```python
from build123d import *

# Parameters (mm, degrees)
SKETCH_1_W               = 27
SKETCH_1_H               = 17
EXTRUDE_1_DEPTH          = 1
SKETCH_2_R               = 2.55
CUT_EXTRUDE_1_DEPTH      = 16.984367363
EXTRUDE_2_DEPTH          = 17
SKETCH_6_W               = 1.5
SKETCH_6_H               = 2
EXTRUDE_3_DEPTH          = 2
CHAMFER_1_SIZE           = 1
CUT_EXTRUDE_4_REACH      = 39.316
SKETCH_8_R               = 2
FILLET_1_R               = 3
SKETCH_9_W               = 7
SKETCH_9_H               = 13
EXTRUDE_4_DEPTH          = 1.5
SKETCH_7_R               = 1.35
CUT_EXTRUDE_5_DEPTH      = 10
CUT_EXTRUDE_6_REACH      = 41.373
FILLET_2_R               = 2.2
SKETCH_13_W              = 11.6
SKETCH_13_H              = 5.4
EXTRUDE_6_DEPTH          = 5.4
CUT_EXTRUDE_7_DEPTH      = 45.299097095
CUT_EXTRUDE_7_DEPTH_BACK = 45.299097095
SKETCH_14_OUTSIDE_W      = 46.85
SKETCH_14_OUTSIDE_H      = 49.25
SKETCH_14_OUTSIDE_W_2    = 27
SKETCH_14_OUTSIDE_H_2    = 6.9
EXTRUDE_7_DEPTH          = 3.5
EXTRUDE_7_DEPTH_BACK     = 10.5
SKETCH_16_W              = 5.6
SKETCH_16_H              = 1.5
SKETCH_16_W_2            = 4.4
SKETCH_16_W_3            = 12.2
EXTRUDE_8_DEPTH          = 2
EXTRUDE_9_DEPTH          = 2.5
CUT_EXTRUDE_8_REACH      = 55.893
SKETCH_18_W              = 5
SKETCH_18_H              = 9
EXTRUDE_START            = -1.5
SKETCH_19_R              = 3.726433752
SKETCH_19_R_2            = 1.35
SKETCH_19_W              = 24.8
SKETCH_19_H              = 1.288897449
EXTRUDE_10_DEPTH         = 1.5
FILLET_4_R               = 2


# Some blends are built 0.0001 mm under size
with BuildPart() as part:
    # 草图1 → 凸台-拉伸1 (new body)
    with BuildSketch(Plane.XY):
        Rectangle(SKETCH_1_W, SKETCH_1_H)
    extrude(amount=EXTRUDE_1_DEPTH)

    # 草图2 → 切除-拉伸1 (cut, through all)
    with BuildSketch(Plane.XY.offset(1)):
        with Locations((0, 4.125)):
            Circle(SKETCH_2_R)
        with Locations((0, -4.125)):
            Circle(SKETCH_2_R)
        with Locations((8.27, 4.125)):
            Circle(SKETCH_2_R)
        with Locations((8.27, -4.125)):
            Circle(SKETCH_2_R)
        with Locations((-8.27, 4.125)):
            Circle(SKETCH_2_R)
        with Locations((-8.27, -4.125)):
            Circle(SKETCH_2_R)
    extrude(amount=-CUT_EXTRUDE_1_DEPTH, mode=Mode.SUBTRACT)

    # 草图3 → 凸台-拉伸2 (add)
    with BuildSketch(Plane.XZ.offset(8.5)):
        Polygon((13.5, 0), (19, 0), (19, -28.5), (-13.5, -28.5), (-13.5, -30), (20.5, -30), (20.5, 1), (13.5, 1), align=None)
    extrude(amount=-EXTRUDE_2_DEPTH)

    # 草图6 → 凸台-拉伸3 (add, symmetric)
    with BuildSketch(Plane(origin=(0, 0, 0), x_dir=(1, 0, 0), z_dir=(0, 1, 0))):
        Polygon((19, 0), (19, 5), (14, 0), align=None)
        Polygon((19, 28.5), (14, 28.5), (19, 23.5), align=None)
        with Locations((18.25, 20)):
            Rectangle(SKETCH_6_W, SKETCH_6_H)
    extrude(amount=EXTRUDE_3_DEPTH, both=True)

    # 倒角1
    chamfer_1_edges = [part.edges().sort_by_distance(p)[0] for p in [
        (-13.5, 0, 0),
    ]]
    chamfer(chamfer_1_edges, length=CHAMFER_1_SIZE - 0.0001)  # a hair under: the kernel refuses the full size

    # 草图8 → 切除-拉伸4 (cut, up to next)
    with BuildSketch(Plane(origin=(0, 0, 0), x_dir=(-1, 0, 0), z_dir=(0, 0, -1)), mode=Mode.PRIVATE) as cut_extrude_4_sk1:
        Circle(SKETCH_8_R)
    cut_extrude_4_tool1 = extrude(cut_extrude_4_sk1.sketch, amount=-CUT_EXTRUDE_4_REACH, mode=Mode.PRIVATE) & part.part
    add(cut_extrude_4_tool1.solids().sort_by_distance((0, 0, 0))[0], mode=Mode.SUBTRACT)

    # 圆角1
    fillet_1_edges = [part.edges().sort_by_distance(p)[0] for p in [
        (20.5, 0, 1),
        (20.5, 0, -30),
        (19, 5.25, -28.5),
        (19, 5.25, 0),
        (19, -5.25, 0),
        (19, -5.25, -28.5),
    ]]
    fillet(fillet_1_edges, radius=FILLET_1_R)

    # 草图9 → 凸台-拉伸4 (add)
    with BuildSketch(Plane(origin=(0, 0, -30), x_dir=(-1, 0, 0), z_dir=(0, 0, -1))):
        with Locations((0, 6.5)):
            Rectangle(SKETCH_9_W, SKETCH_9_H)
    extrude(amount=-EXTRUDE_4_DEPTH)

    # 草图7 → 切除-拉伸5 (cut)
    with BuildSketch(Plane(origin=(0, 0, -30), x_dir=(-1, 0, 0), z_dir=(0, 0, -1))):
        with Locations((0, 10)):
            Circle(SKETCH_7_R)
        with Locations((-8.5, 2.7)):
            Circle(SKETCH_7_R)
        with Locations((8.5, 2.7)):
            Circle(SKETCH_7_R)
    extrude(amount=-CUT_EXTRUDE_5_DEPTH, mode=Mode.SUBTRACT)

    # 草图11 → 切除-拉伸6 (cut, up to next)
    with BuildSketch(Plane(origin=(0, 0, -30), x_dir=(-1, 0, 0), z_dir=(0, 0, -1)), mode=Mode.PRIVATE) as cut_extrude_6_sk1:
        with BuildLine():
            Line((13.5, -8.5), (13.5, 0))
            Line((13.5, 0), (-9, 0))
            ThreePointArc((-9, 0), (-15.01040764, -2.48959236), (-17.5, -8.5))
            Line((-17.5, -8.5), (13.5, -8.5))
        make_face()
    cut_extrude_6_tool1 = extrude(cut_extrude_6_sk1.sketch, amount=-CUT_EXTRUDE_6_REACH, mode=Mode.PRIVATE) & part.part
    add(cut_extrude_6_tool1.solids().sort_by_distance((1.149624, -4.397011, -30))[0], mode=Mode.SUBTRACT)

    # 圆角2
    fillet_2_edges = [part.edges().sort_by_distance(p)[0] for p in [
        (-3.5, 13, -29.25),
        (-3.5, 8.5, -29.25),
        (3.5, 13, -29.25),
        (3.5, 8.5, -29.25),
        (-13.5, 0, -29.25),
        (-13.5, 8.5, -29.25),
    ]]
    fillet(fillet_2_edges, radius=FILLET_2_R)

    # 草图13 → 凸台-拉伸6 (add)
    with BuildSketch(Plane(origin=(0, 0, -30), x_dir=(-1, 0, 0), z_dir=(0, 0, -1))):
        with Locations((0, 2.7)):
            Rectangle(SKETCH_13_W, SKETCH_13_H)
    extrude(amount=EXTRUDE_6_DEPTH)

    # 草图14 outside → 切除-拉伸7 (cut, two sides: drawn at the far end of the back side and taken through both)
    with BuildSketch(Plane(origin=(0, 8.5, 0), x_dir=(1, 0, 0), z_dir=(0, 1, 0)).offset(-CUT_EXTRUDE_7_DEPTH_BACK)):
        with Locations((3.5, 17.2)):
            Rectangle(SKETCH_14_OUTSIDE_W, SKETCH_14_OUTSIDE_H)
        with Locations((0, 31.95)):
            Rectangle(SKETCH_14_OUTSIDE_W_2, SKETCH_14_OUTSIDE_H_2, mode=Mode.SUBTRACT)
    extrude(amount=CUT_EXTRUDE_7_DEPTH + CUT_EXTRUDE_7_DEPTH_BACK, mode=Mode.SUBTRACT)

    # 草图15 → 凸台-拉伸7 (add, two sides: drawn at the far end of the back side and taken through both)
    with BuildSketch(Plane.XZ.offset(-EXTRUDE_7_DEPTH_BACK)):
        Polygon((-19.25, -14.25), (-19.25, -30), (-11.3, -30), (-11.3, -28.5), (-17.75, -28.5), (-17.75, -19.35), (-16.15, -19.35), (-16.15, -17.35), (-17.75, -17.35), (-17.75, -16.25), (-15.25, -16.25), (-15.25, -14.25), align=None)
        Polygon((17.75, -28.5), (13.5, -28.5), (13.5, -30), (19.25, -30), (19.25, -14.25), (15.25, -14.25), (15.25, -16.25), (17.75, -16.25), (17.75, -17.35), (16.15, -17.35), (16.15, -19.35), (17.75, -19.35), align=None)
    extrude(amount=EXTRUDE_7_DEPTH + EXTRUDE_7_DEPTH_BACK)

    # 草图16 → 凸台-拉伸8 (add)
    with BuildSketch(Plane(origin=(0, 8.5, 0), x_dir=(1, 0, 0), z_dir=(0, 1, 0))):
        with Locations((-8.5, 29.25)):
            Rectangle(SKETCH_16_W, SKETCH_16_H)
        with Locations((-3.5, 29.25)):
            Rectangle(SKETCH_16_W_2, SKETCH_16_H)
        with Locations((7.4, 29.25)):
            Rectangle(SKETCH_16_W_3, SKETCH_16_H)
    extrude(amount=EXTRUDE_8_DEPTH)

    # 草图17 → 凸台-拉伸9 (add, symmetric)
    with BuildSketch(Plane(origin=(0, 3.5, 0), x_dir=(-1, 0, 0), z_dir=(0, -1, 0))):
        Polygon((17.75, 25.275), (14.525, 28.5), (17.75, 28.5), align=None)
        Polygon((-17.75, 25.275), (-17.75, 28.5), (-14.525, 28.5), align=None)
    extrude(amount=EXTRUDE_9_DEPTH, both=True)

    # 草图18 → 切除-拉伸8 (cut, up to next)
    with BuildSketch(Plane.ZY.offset(19.25), mode=Mode.PRIVATE) as cut_extrude_8_sk1:
        with Locations((-19.85, 3.5)):
            Rectangle(SKETCH_18_W, SKETCH_18_H)
    cut_extrude_8_tool1 = extrude(cut_extrude_8_sk1.sketch, amount=-CUT_EXTRUDE_8_REACH, mode=Mode.PRIVATE) & part.part
    add(cut_extrude_8_tool1.solids().sort_by_distance((-19.25, 3.5, -19.85))[0], mode=Mode.SUBTRACT)

    # 草图19 → 凸台-拉伸10 (add)
    # profile 1 of 2: a face of its own
    with BuildSketch(Plane.XY.offset(-28.5).offset(EXTRUDE_START)):
        with Locations((0, 10)):
            Circle(SKETCH_19_R)
        with Locations((0, 10)):
            Circle(SKETCH_19_R_2, mode=Mode.SUBTRACT)
    # profile 2 of 2: a face of its own
    with BuildSketch(Plane.XY.offset(-28.5).offset(EXTRUDE_START)):
        with Locations((1.1, -0.644448725)):
            Rectangle(SKETCH_19_W, SKETCH_19_H)
    extrude(amount=EXTRUDE_10_DEPTH)

    # 圆角4
    # the kernel refuses this fillet: 2 mm, written as the material it adds along each edge
    with BuildSketch(Plane(origin=(-5.8, 5.4, -30), x_dir=(0, 1, 0), z_dir=(1, 0, 0))) as fillet_4_piece_1:
        with BuildLine():
            CenterArc((FILLET_4_R, -FILLET_4_R), FILLET_4_R, 90, 90)
            Line((0, -FILLET_4_R), (0, 0))
            Line((0, 0), (FILLET_4_R, 0))
        make_face()
    extrude(amount=11.6)
    with BuildSketch(Plane(origin=(13.5, -1.288897449, -28.5), x_dir=(0, -1, 0), z_dir=(0, 0, -1))) as fillet_4_piece_2:
        with BuildLine():
            CenterArc((FILLET_4_R, FILLET_4_R), FILLET_4_R, 180, 90)
            Line((0, FILLET_4_R), (0, 0))
            Line((0, 0), (FILLET_4_R, 0))
        make_face()
    extrude(amount=1.5)
    with BuildSketch(Plane(origin=(17.75, 1, -28.5), x_dir=(-1, 0, 0), z_dir=(0, 1, 0)), Plane(origin=(-17.75, 6, -28.5), x_dir=(1, 0, 0), z_dir=(0, -1, 0)), Plane(origin=(-17.75, 10.5, -28.5), x_dir=(1, 0, 0), z_dir=(0, -1, 0)), Plane(origin=(17.75, -3.5, -28.5), x_dir=(-1, 0, 0), z_dir=(0, 1, 0))) as fillet_4_piece_3:
        with BuildLine():
            CenterArc((FILLET_4_R, FILLET_4_R), FILLET_4_R, 180, 90)
            Line((0, FILLET_4_R), (0, 0))
            Line((0, 0), (FILLET_4_R, 0))
        make_face()
    extrude(amount=9.5)
    with BuildSketch(Plane(origin=(-3.692737265, 10.5, -28.5), x_dir=(-1, 0, 0), z_dir=(0, 0, -1))) as fillet_4_piece_4:
        with BuildLine():
            CenterArc((1.459159814, 2), FILLET_4_R, 205.88535786, 64.11464214)
            ThreePointArc((-0.340178937, 1.126856222), (-0.125315404, 0.576944648), (0, 0))
            Line((0, 0), (1.459159814, 0))
        make_face()
    extrude(amount=1.5)
    with BuildSketch(Plane(origin=(3.692737265, 10.5, -28.5), x_dir=(-0.28900142054358374, 0.9573286681823493, 0), z_dir=(0, 0, -1))) as fillet_4_piece_5:
        with BuildLine():
            CenterArc((1.492958077, 1.974898363), FILLET_4_R, 196.798181975, 64.11464214)
            Line((-0.421699259, 1.396895522), (0, 0))
            ThreePointArc((0, 0), (0.588541981, 0.046769794), (1.177083962, 0))
        make_face()
    extrude(amount=1.5)
    with BuildSketch(Plane(origin=(-5.8, 0, -30), x_dir=(0, -1, 0), z_dir=(1, 0, 0))) as fillet_4_piece_6:
        with BuildLine():
            CenterArc((2, 1.869313554), FILLET_4_R, 180, 69.172765444)
            Line((0, 1.869313554), (0, 0))
            Line((0, 0), (1.288897449, 0))
        make_face()
    extrude(amount=11.6)
    with BuildSketch(Plane(origin=(-11.3, -1.288897449, -30), x_dir=(1, 0, 0), z_dir=(0, 0, 1))) as fillet_4_piece_7:
        with BuildLine():
            CenterArc((FILLET_4_R, -FILLET_4_R), FILLET_4_R, 90, 90)
            Line((0, -FILLET_4_R), (0, 0))
            Line((0, 0), (FILLET_4_R, 0))
        make_face()
    extrude(amount=1.5)
    # the kernel refuses this fillet: 2 mm, written as the material it takes off along each edge
    with BuildSketch(Plane(origin=(19.25, 15.5, -30), x_dir=(-1, 0, 0), z_dir=(0, -1, 0))) as fillet_4_2_piece_1:
        with BuildLine():
            CenterArc((FILLET_4_R, -FILLET_4_R), FILLET_4_R, 90, 90)
            Line((0, -FILLET_4_R), (0, 0))
            Line((0, 0), (FILLET_4_R, 0))
        make_face()
    extrude(amount=24, mode=Mode.SUBTRACT)
    with BuildSketch(Plane(origin=(-19.25, 15.5, -30), x_dir=(1, 0, 0), z_dir=(0, -1, 0))) as fillet_4_2_piece_2:
        with BuildLine():
            CenterArc((FILLET_4_R, FILLET_4_R), FILLET_4_R, 180, 90)
            Line((0, FILLET_4_R), (0, 0))
            Line((0, 0), (FILLET_4_R, 0))
        make_face()
    extrude(amount=24, mode=Mode.SUBTRACT)


solid = part.part
```
Geometry: final body of the model. Coordinates: model frame, mm. A direction names the side the tool comes from. Coordinates: 2 decimals unless noted, no trailing zeros. Order: outer loops, then holes, each group sorted by start corner. A loop starts at its lowest first (then second) coordinate and runs counter-clockwise, first axis right, second up. Notation, with made-up numbers: (16.5, 53) -> (62.5, 53) arc R23 cw to (62.5, 86) -> close; hole circle Ø5 at (-6.5, -14.5). An arc over 180 degrees is marked (long way). Write each question's results on one line, items separated by ' | '. Start each with the question number.
1) First-contact query: pin 1 (2.5 mm diameter, centred on x = -17.5, z = -20, fed in from +Y); pin 2 (1 mm diameter, centred on x = -0.5, z = -33, fed in from +Y); pin 3 (1.8 mm diameter, centred on x = -16.5, y = -3, fed in from -Z). Flat tips, straight axial feed; report the tip coordinate or a pass-through.
2) Mould query, pull axis Z, two halves, no side actions, for faces 1 (the flat face through (17.75, 4, -23)), 2 (the flat face through (-4, 9, -30)), 3 (the cylindrical face through (4.1, 10.8, -29.2)). Classes: released by +Z, released by -Z, zero draft, split by the parting line, or undercut.
3) Set-up query: faces 4 (the flat face through (-18, 8, -19)), 5 (the flat face through (0, 5.4, -34)), 6 (the flat face through (16.5, 1, -27.3)), 7 (the flat face through (15.25, 4, -15)), 8 (the flat face through (17, 4, -17.35)). Return all of +Z, -Z, +X, -X, +Y, -Y with unobstructed straight access to the full face (end or side cutting, diameter ignored); none if empty.
4) Cut plane B-B, the plane z = -23. Output: boundary loops of the cut face in (x, y), and give its area (3 significant figures).
5) Cut plane A-A, the plane x = 0. Output: boundary loops of the cut face in (y, z).
6) Cut plane C-C, the plane y = 2.7. State how many separate pieces and enclosed holes the cut face has, and give its area (3 significant figures).
7) Material intervals for line 1 along Y through (x, z) = (8.5, -28.95); line 2 along X through (y, z) = (9, -16); line 3 along X through (y, z) = (-0.75, -16.75), sorted ascending.
8) Cut plane D-D, the plane x = 8.5. Output: boundary loops of the cut face in (y, z).
Checks:
1) pin 1: y = 10.5 | pin 2: y = 5.4 | pin 3: z = -30
2) face 1: undercut | face 2: released by -Z | face 3: zero draft
3) face 4: -X | face 5: -Z, +X, -X, +Y | face 6: -Y | face 7: +Z, +Y, -Y | face 8: +Y, -Y
4) outline: (-19.25, -3.5) -> (-17.75, -3.5) -> (-17.75, 10.5) -> (-19.25, 10.5) -> close; (17.75, -3.5) -> (19.25, -3.5) -> (19.25, 10.5) -> (17.75, 10.5) -> close | area: 42.0 mm^2
5) outline: (-1.29, -30) arc R2 cw to (0, -31.87) -> (0, -35.4) -> (5.4, -35.4) -> (5.4, -32) arc R2 cw to (7.4, -30) -> (8.65, -30) -> (8.65, -28.5) -> (-1.29, -28.5) -> close; (11.35, -30) -> (13.73, -30) -> (13.73, -28.5) -> (11.35, -28.5) -> close
6) separate pieces: 4 | enclosed holes: 0 | area: 169 mm^2
7) line 1: -1.29 to 1.35, 4.05 to 10.5 | line 2: -19.25 to -15.25, 15.25 to 19.25 | line 3: -19.25 to -17.75, 17.75 to 19.25
8) outline: (-1.29, -30) -> (1.35, -30) -> (1.35, -28.5) -> (-1.29, -28.5) -> close; (4.05, -30) -> (10.5, -30) -> (10.5, -28.5) -> (4.05, -28.5) -> close
